from build123d import *

# Parameters (mm, degrees)
EXTRUDE_THIN1_DEPTH = 10
SKETCH3_W           = 9.525
SKETCH3_H           = 9.525
BOSS_EXTRUDE1_DEPTH = 10
SKETCH4_W           = 25.457542158
SKETCH4_H           = 16.944951572
CUT_EXTRUDE1_DEPTH  = 12.917655
SKETCH5_W           = 71.291664715
SKETCH5_H           = 18.17592298
CUT_EXTRUDE2_DEPTH  = 12.917655


# Read off the part's stored shape, not the designer's step: Extrude-Thin1
with BuildPart() as part:
    # Extrude-Thin1 outline → Extrude-Thin1 (new body)
    with BuildSketch(Plane(origin=(9.525, 0, 0), x_dir=(0, 0, -1), z_dir=(1, 0, 0))):
        Polygon((-323.6, 99.7625), (-323.6, 95), (-326.426404213, 98.833124766), (-466.921154801, -4.7625), (9.721154801, -4.7625), (-130.773595787, 98.833124766), (-133.6, 95), (-133.6, 99.7625), align=None)
        Polygon((-276.860305191, 4.7625), (-437.953845199, 4.7625), (-325.055829502, 88.009314718), align=None, mode=Mode.SUBTRACT)
        Polygon((-180.339694809, 4.7625), (-132.144170498, 88.009314718), (-19.246154801, 4.7625), align=None, mode=Mode.SUBTRACT)
        Polygon((-315.339694809, 90.2375), (-233.3625, 90.2375), (-233.3625, 4.7625), (-265.854168493, 4.7625), align=None, mode=Mode.SUBTRACT)
        Polygon((-223.8375, 90.2375), (-141.860305191, 90.2375), (-191.345831507, 4.7625), (-223.8375, 4.7625), align=None, mode=Mode.SUBTRACT)
    extrude(amount=EXTRUDE_THIN1_DEPTH)

    # Sketch3 → Boss-Extrude1 (add)
    with BuildSketch(Plane(origin=(19.525, 0, 0), x_dir=(0, 0, -1), z_dir=(1, 0, 0))):
        Polygon((-133.6, 99.7625), (-133.6, 95), (-130.773595787, 98.833124766), (-132.033999804, 99.7625), align=None)
        Polygon((-326.426404213, 98.833124766), (-323.6, 95), (-323.6, 99.7625), (-325.166000196, 99.7625), align=None)
        Polygon((9.721154801, 4.7625), (-3.196499804, 4.7625), (9.721154801, -4.7625), align=None)
        Polygon((-466.921154801, -4.7625), (-454.003500196, 4.7625), (-466.921154801, 4.7625), align=None)
        with Locations((-260.802793514, 9.525)):
            Rectangle(SKETCH3_W, SKETCH3_H)
        with Locations((-196.397206486, 9.525)):
            Rectangle(SKETCH3_W, SKETCH3_H)
    extrude(amount=-BOSS_EXTRUDE1_DEPTH)

    # Sketch4 → Cut-Extrude1 (cut)
    with BuildSketch(Plane(origin=(0, 0, -9.721154801), x_dir=(-1, 0, 0), z_dir=(0, 0, -1))):
        with Locations((-19.165581616, -1.578540654)):
            Rectangle(SKETCH4_W, SKETCH4_H)
    extrude(amount=-CUT_EXTRUDE1_DEPTH, mode=Mode.SUBTRACT)

    # Sketch5 → Cut-Extrude2 (cut)
    with BuildSketch(Plane.XY.offset(466.921154801)):
        with Locations((18.052286902, -0.452774422)):
            Rectangle(SKETCH5_W, SKETCH5_H)
    extrude(amount=-CUT_EXTRUDE2_DEPTH, mode=Mode.SUBTRACT)


solid = part.part
Input: part model. Units: mm. Frame: model coordinates. A direction names the side the tool comes from. Give positions to 0.01 mm unless a question says otherwise; leave off trailing zeros. Loops run counter-clockwise (first coordinate to the right, second up) from the corner with the lowest first, then second, coordinate; pieces in that order, holes last. Notation, with made-up numbers: M 72,-32.5 L 102,-32.5 A7 cw 102,-20.5 Z; hole C -14.75,37.5 d11. An arc over 180 degrees is marked long. Use one line per item in the form item = value.
1. Section query A-A, the plane x = 14.5. Return the cut outline in (y, z), and give its area (3 significant figures).
Numbers:
outline = M -4.76,3.2 L 4.76,3.2 L 99.76,132.03 L 99.76,325.17 L 4.76,454 L -4.76,454 Z; hole M 4.76,19.25 L 88.01,132.14 L 4.76,180.34 Z; hole M 4.76,191.35 L 90.24,141.86 L 90.24,223.84 L 4.76,223.84 L 4.76,201.16 L 14.29,201.16 L 14.29,191.63 L 4.76,191.63 Z; hole M 4.76,233.36 L 90.24,233.36 L 90.24,315.34 L 4.76,265.85 L 4.76,265.57 L 14.29,265.57 L 14.29,256.04 L 4.76,256.04 Z; hole M 4.76,276.86 L 88.01,325.06 L 4.76,437.95 Z
area = 11,900 mm²
2. Section query B-B, the plane z = 74. Return the cut outline in (x, y) (1 decimal), and give its area (3 significant figures).
Numbers:
outline = M 9.5,-4.8 L 19.5,-4.8 L 19.5,4.8 L 9.5,4.8 Z; M 9.5,45.1 L 19.5,45.1 L 19.5,57 L 9.5,57 Z
area = 214 mm²
3. Reachability of faces 5 (the face through (14.5, 45.8, 382.3)), 6 (the face through (14, 0, 454.003)) from +Z, -Z, +X, -X, +Y, -Y: full face, straight path, thin tool, end or side. Return the list, or none.
Numbers:
face_5 = +X, -X
face_6 = +Z, +X, -X, +Y, -Y
4. Pull-direction query (Y, two-part tool) for faces 1 (the face through (15, 0, 3.197)), 2 (the face through (15, 99.762, 227)), 3 (the face through (14, 4.762, 99)), 4 (the face through (14.455, 48.098, 166.257)); classes: released by +Y, released by -Y, zero draft, split by the parting line, or undercut.
Numbers:
face_1 = zero draft
face_2 = released by +Y
face_3 = undercut
face_4 = undercut
5. First-contact query: pin 1 (5 mm diameter, centred on x = 17, y = 34, fed in from +Z); pin 2 (3 mm diameter, centred on x = 15, z = 115, fed in from +Y); pin 3 (2 mm diameter, centred on x = 13, y = 70, fed in from +Z). Flat tips, straight axial feed; report the tip coordinate or a pass-through.
Numbers:
pin_1 = 417.74
pin_2 = 88.31
pin_3 = 366.89
6. Section query C-C, the plane y = 65.5. Return the cut outline in (x, z) (1 decimal), and give its area (3 significant figures).
Numbers:
outline = M 9.5,85.6 L 19.5,85.6 L 19.5,101.6 L 9.5,101.6 Z; M 9.5,145.2 L 19.5,145.2 L 19.5,156.2 L 9.5,156.2 Z; M 9.5,223.8 L 19.5,223.8 L 19.5,233.4 L 9.5,233.4 Z; M 9.5,301 L 19.5,301 L 19.5,312 L 9.5,312 Z; M 9.5,355.6 L 19.5,355.6 L 19.5,371.6 L 9.5,371.6 Z
area = 636 mm²
7. Line query: L1, parallel to Y at x = 13.5, z = 255.5; L2, parallel to Z at x = 12.5, y = 67; L3, parallel to Y at x = 12.75, z = 152. Output: solid intervals per line, ascending.
Numbers:
L1 = -4.76 to 4.76, 90.24 to 99.76
L2 = 87.6 to 103.65, 144.31 to 155.31, 223.84 to 233.36, 301.89 to 312.89, 353.55 to 369.6
L3 = -4.76 to 4.76, 53.71 to 72.72, 90.24 to 99.76
